Answer from the drawing. Dimensions are ordinates in mm from the lowest x, y and z of the part. Coordinates: 2 decimals unless noted, no trailing zeros. Write each loop counter-clockwise with the first axis right and the second up, starting at its lowest first coordinate (ties: lowest second). Pieces come first, ordered by that corner, then holes. Notation, with made-up numbers: (43.25, 9.5) - (79.25, 9.5) arc R29 cw to (79.25, 30.5) - close; hole circle Ø6 at (60, 48.25). An arc over 180 degrees is marked (long way). Use a Markdown table: item, result.
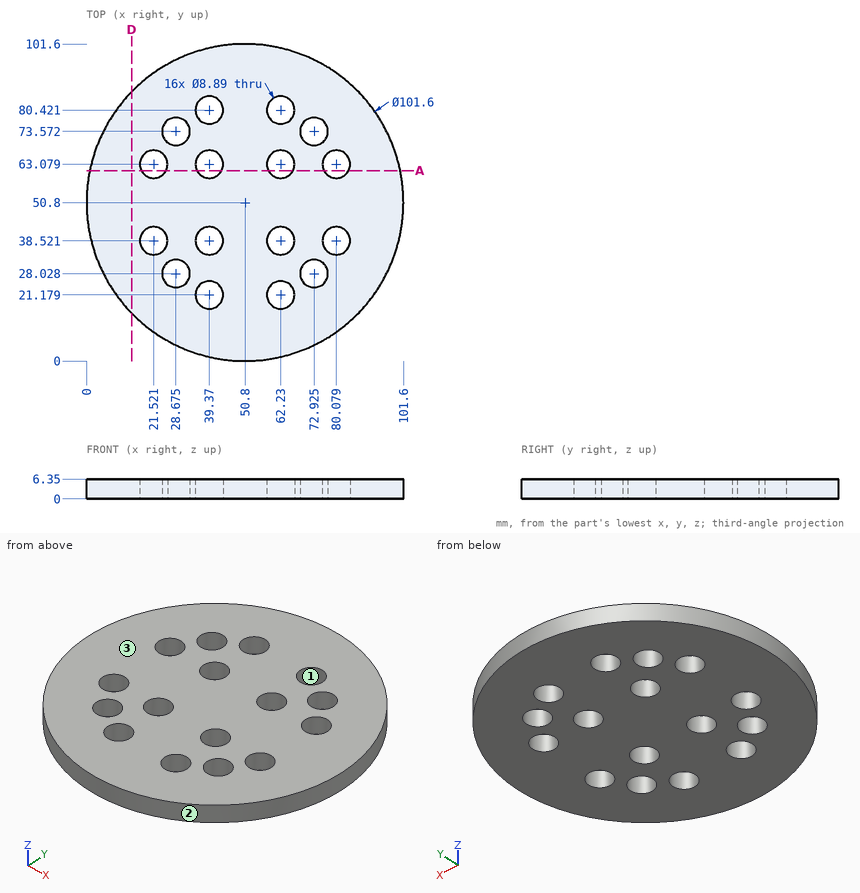
(1) The mould has two halves that part along X. Classify the marked faces 1, 2 and 3: pulls with the +X half, pulls with the -X half, needs draft (parallel to the pull), parting line crosses it, or undercut.
Report:
| item | result |
|---|---|
| face 1 | undercut |
| face 2 | parting line crosses it |
| face 3 | needs draft |
(2) A cutting plane is placed at D-D, the plane x = 14.5. Write down the section's boundary in (y, z).
Report:
| item | result |
|---|---|
| outline | (15.26, 0) - (86.34, 0) - (86.34, 6.35) - (15.26, 6.35) - close |
(3) Straight lines are drawn through the part: L1, parallel to Y at x = 39.5, z = 3.75 (1 decimal); L2, parallel to Y at x = 28, z = 0.5 (1 decimal); L3, parallel to Y at x = 32.5, z = 3.5 (1 decimal). For each, find the intervals that lie inside material, in ascending order.
Report:
| item | result |
|---|---|
| L1 | y = 1.3 to 16.7, 25.6 to 34.1, 43 to 58.6, 67.5 to 76, 84.9 to 100.3 |
| L2 | y = 5.4 to 23.6, 32.4 to 69.2, 78 to 96.2 |
| L3 | y = 3.4 to 25.8, 30.3 to 71.3, 75.8 to 98.2 |
(4) Each of these flat-tipped pins is pushed along its axis until it touches: P1, Ø7, axis at x = 39.37, y = 80.42, coming from the +Z side; P2, Ø10, axis at x = 80.5, y = 86, coming from the -Z side; P3, Ø1, axis at y = 47, z = 0.5, coming from the -X side. Where does it stop, or does it pass through?
Report:
| item | result |
|---|---|
| P1 | passes through |
| P2 | stops at z = 0 |
| P3 | stops at x = 0.11 |
(5) A cutting plane is placed at A-A, the plane y = 61. Count the separate pieces of the cut face and the enclosed holes in it.
Report:
| item | result |
|---|---|
| separate pieces | 5 |
| enclosed holes | 0 |
